CAD build for the part. Positions are in the model's coordinates, mm. Face numbers are marked on the shaded views. A direction names the side the tool comes from. Give positions to 0.01 mm unless a question says otherwise; leave off trailing zeros. Write each loop counter-clockwise with the first axis right and the second up, starting at its lowest first coordinate (ties: lowest second). Pieces come first, ordered by that corner, then holes. Notation, with made-up numbers: (13, 83.25) - (57, 83.25) arc R18 ccw to (57, 118.25) - close; hole circle Ø4 at (-14, 83.25). An arc over 180 degrees is marked (long way). Put each result on its own line as item: value. Start each with the question number.
1. Cut at A-A on x = 0. List the corners of the cut face in (y, z), and give its area (3 significant figures).
2. Cut at D-D on y = 26. List the corners of the cut face in (x, z).
3. Cut at C-C on z = 1.7. List the corners of the cut face in (x, y), and give its area (3 significant figures).
4. Wall check: line 1 (X direction, y = 0.5, z = 1.3); line 2 (Z direction, x = 17.5, y = -15); line 3 (X direction, y = -8.5, z = 1.8). Give the ranges that are in metal, low to high.
5. Tool access for the marked faces 1 and 2: list every direction of +Z, -Z, +X, -X, +Y, -Y with a clear straight run to the whole face (end or side of a thin tool).
6. Drop flat-ended pins along their axis: pin 1 (2 mm diameter, centred on x = -19, y = -6, fed in from -Z); pin 2 (1 mm diameter, centred on x = -1, z = 0.5, fed in from -Y); pin 3 (1 mm diameter, centred on y = 2, z = 1, fed in from -X); pin 4 (1 mm diameter, centred on x = -3.5, z = 1, fed in from +Y). Give the stop position or say it passes through.
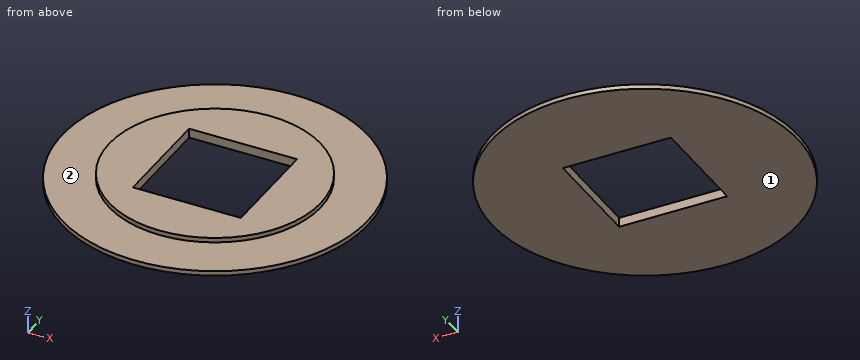
Autodesk Fusion 360 part; units mm, degrees
sketch "Sketch1" plane through (0, 0, 0) normal (0, 0, 1) x (1, 0, 0)
  circle A0 centre (0, 0) radius 32.5
  line L0 (-11.5, 11.5) -> (11.5, 11.5)
  line L1 (11.5, 11.5) -> (11.5, -11.5)
  line L2 (11.5, -11.5) -> (-11.5, -11.5)
  line L3 (-11.5, -11.5) -> (-11.5, 11.5)
  point P0 (11.5, 0)
  point P1 (0, 11.5)
  dimension "d1" = 65
  dimension "d2" = 23
extrude "Extrude1" add sketch "Sketch1" along normal blind 1
sketch "Sketch2" plane through (0, 0, 1) normal (0, 0, 1) x (-1, 0, 0)
  line L0 (-11.5, 11.5) -> (11.5, 11.5)
  line L1 (11.5, 11.5) -> (11.5, -11.5)
  line L2 (11.5, -11.5) -> (-11.5, -11.5)
  line L3 (-11.5, -11.5) -> (-11.5, 11.5)
  circle A0 centre (0, 0) radius 32.5
  line L4 (11.5, -11.5) -> (-11.5, -11.5)
  line L5 (-11.5, -11.5) -> (-11.5, 11.5)
  line L6 (-11.5, 11.5) -> (11.5, 11.5)
  line L7 (11.5, 11.5) -> (11.5, -11.5)
  circle A1 centre (0, 0) radius 22.5
  dimension "d5" = 45
extrude "Extrude2" add sketch "Sketch2" along normal blind 1 contours A1
Report:
1. outline: (-32.5, 0) - (-11.5, 0) - (-11.5, 2) - (-22.5, 2) - (-22.5, 1) - (-32.5, 1) - close; (11.5, 0) - (32.5, 0) - (32.5, 1) - (22.5, 1) - (22.5, 2) - (11.5, 2) - close
1. area: 64.0 mm²
2. outline: (-19.5, 0) - (19.5, 0) - (19.5, 1) - (-19.5, 1) - close
3. outline: circle Ø45 at (0, 0); hole (-11.5, -11.5) - (11.5, -11.5) - (11.5, 11.5) - (-11.5, 11.5) - close
3. area: 1,060 mm²
4. line 1: x = -22.49 to -11.5, 11.5 to 22.49
4. line 2: z = 0 to 1
4. line 3: x = -20.83 to -11.5, 11.5 to 20.83
5. face 1: -Z, +X, -X, +Y, -Y
5. face 2: +Z
6. pin 1: stops at z = 0
6. pin 2: stops at y = -32.5
6. pin 3: stops at x = -32.47
6. pin 4: stops at y = 32.36
